```python
from build123d import *

# Parameters (mm, degrees)
F0_R     = 3.175
F1_DEPTH = 76.2
F2_R     = 1.27
F3_DEPTH = 3.176
F4_DEPTH = 3.176


with BuildPart() as f1:
    # F0 (on Front) → F1 (new body)
    with BuildSketch(Plane.XZ):
        Circle(F0_R)
    extrude(amount=-F1_DEPTH)

    # F2 (on Right) → F3 (cut, through all)
    with BuildSketch(Plane.YZ):
        with Locations((2.54, 0)):
            Circle(F2_R)
        with Locations((73.66, 0)):
            Circle(F2_R)
    extrude(amount=F3_DEPTH, mode=Mode.SUBTRACT)

    # F2 (on Right) → F4 (cut, through all)
    with BuildSketch(Plane.YZ):
        with Locations((2.54, 0)):
            Circle(F2_R)
        with Locations((73.66, 0)):
            Circle(F2_R)
    extrude(amount=-F4_DEPTH, mode=Mode.SUBTRACT)


solid = f1.part
```
The listing builds one solid part. Answer for the finished solid, in the listing's coordinates (mm). Give positions to 0.01 mm unless a question says otherwise; leave off trailing zeros. Order: outer loops, then holes, each group sorted by start corner. A loop starts at its lowest first (then second) coordinate and runs counter-clockwise, first axis right, second up. Notation, with made-up numbers: (-8.75, 72) - (12.25, 72) arc R5 ccw to (12.25, 77) - close; hole circle Ø6 at (-3, 75). An arc over 180 degrees is marked (long way). Answer in a Markdown table with one row per item. Add a question column.
Q1. Find the intervals of material crossed by line 1 along Y through (x, z) = (2.2, 0); line 2 along Z through (x, y) = (-0.25, 67.5); line 3 along Y through (x, z) = (0.25, 1), in increasing order. Write a range as [from, to].
Q2. Given P1, Ø1, axis at y = 42, z = -1, coming from the -X side, flat-ended and moving along its own axis, determine where the tip first touches the part or whether it passes through.
Q3. The part is cut by section B-B (x = 1.5). Determine the outline of the cut face in (y, z).
Q4. The part is cut by section C-C (y = 2.54). Determine the outline of the cut face in (x, z) (3 decimals), then the cut area to 3 significant figures.
Q5. The part is cut by section A-A (z = 0). Determine the outline of the cut face in (x, y) (3 decimals), then the cut area to 3 significant figures.
Q6. The part is cut by section D-D (y = 11). Determine the outline of the cut face in (x, z) (3 decimals), then the cut area to 3 significant figures.
Determined:
| question | item | result |
|---|---|---|
| 1 | line 1 | y = [0, 1.27], [3.81, 72.39], [74.93, 76.2] |
| 1 | line 2 | z = [-3.17, 3.17] |
| 1 | line 3 | y = [0, 1.76], [3.32, 72.88], [74.44, 76.2] |
| 2 | P1 | stops at x = -3.14 |
| 3 | outline | (0, -2.8) - (76.2, -2.8) - (76.2, 2.8) - (0, 2.8) - close; hole circle Ø2.54 at (2.54, 0); hole circle Ø2.54 at (73.66, 0) |
| 4 | outline | (-2.91, -1.27) arc R3.175 ccw to (2.91, -1.27) - close; (-2.91, 1.27) - (2.91, 1.27) arc R3.175 ccw to start |
| 4 | area | 16.0 mm² |
| 5 | outline | (-3.175, 0) - (3.175, 0) - (3.175, 1.27) - (-3.175, 1.27) - close; (-3.175, 3.81) - (3.175, 3.81) - (3.175, 72.39) - (-3.175, 72.39) - close; (-3.175, 74.93) - (3.175, 74.93) - (3.175, 76.2) - (-3.175, 76.2) - close |
| 5 | area | 452 mm² |
| 6 | outline | circle Ø6.35 at (0, 0) |
| 6 | area | 31.7 mm² |
